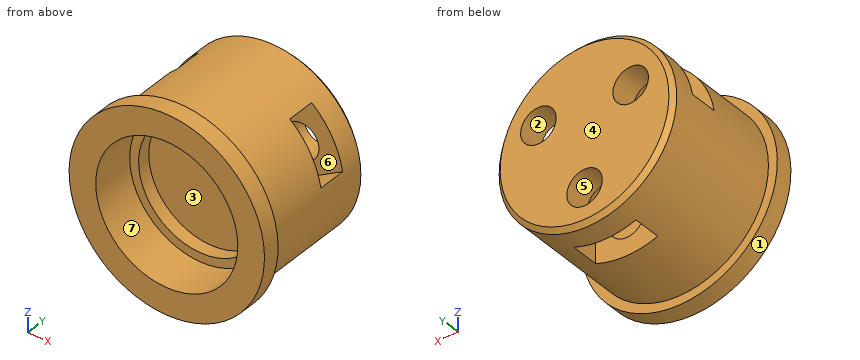
from build123d import *

# Parameters (mm, degrees)
SKETCH1_R           = 10
BOSS_EXTRUDE1_DEPTH = 16
SKETCH2_R           = 11
SKETCH2_R_2         = 10
BOSS_EXTRUDE2_DEPTH = 2
SKETCH3_R           = 8
CUT_EXTRUDE1_DEPTH  = 6.5
SKETCH4_R           = 2
CUT_EXTRUDE2_DEPTH  = 6.5
CUT_EXTRUDE3_START  = -3
SKETCH5_R           = 2
CUT_EXTRUDE3_DEPTH  = 3.2
BOSS_EXTRUDE3_START = -5
SKETCH6_R           = 8
SKETCH6_R_2         = 7
BOSS_EXTRUDE3_DEPTH = 1.5
CHAMFER1_SIZE       = 0.5


with BuildPart() as part:
    # Sketch1 → Boss-Extrude1 (new body)
    with BuildSketch(Plane(origin=(0, 0, 0), x_dir=(1, 0, 0), z_dir=(0, 1, 0))):
        with Locations(Location((0, 0, 0), (0, 0, 270))):
            Circle(SKETCH1_R)
    extrude(amount=BOSS_EXTRUDE1_DEPTH)

    # Sketch2 → Boss-Extrude2 (add)
    with BuildSketch(Plane.XZ):
        with Locations(Location((0, 0, 0), (0, 0, 270))):
            Circle(SKETCH2_R)
        with Locations(Location((0, 0, 0), (0, 0, 270))):
            Circle(SKETCH2_R_2, mode=Mode.SUBTRACT)
    extrude(amount=-BOSS_EXTRUDE2_DEPTH)

    # Sketch3 → Cut-Extrude1 (cut)
    with BuildSketch(Plane.XZ):
        with Locations(Location((0, 0, 0), (0, 0, 270))):
            Circle(SKETCH3_R)
    extrude(amount=-CUT_EXTRUDE1_DEPTH, mode=Mode.SUBTRACT)

    # Sketch4 → Cut-Extrude2 (cut)
    with BuildSketch(Plane(origin=(0, 16, 0), x_dir=(1, 0, 0), z_dir=(0, 1, 0))):
        with Locations(Location((0, 6, 0), (0, 0, 270))):
            Circle(SKETCH4_R)
        with Locations(Location((5.196152423, -3, 0), (0, 0, 270))):
            Circle(SKETCH4_R)
        with Locations(Location((-5.196152423, -3, 0), (0, 0, 270))):
            Circle(SKETCH4_R)
    extrude(amount=-CUT_EXTRUDE2_DEPTH, mode=Mode.SUBTRACT)

    # Sketch5 → Cut-Extrude3 (cut)
    # profile 1 of 3: a face of its own
    with BuildSketch(Plane(origin=(0, 16, 0), x_dir=(1, 0, 0), z_dir=(0, 1, 0)).offset(CUT_EXTRUDE3_START)):
        with BuildLine():
            Line((-3.5, 9.367496998), (-3.5, 3.979274058))
            Line((-3.5, 3.979274058), (0, 1.958548116))
            Line((0, 1.958548116), (3.5, 3.979274058))
            Line((3.5, 3.979274058), (3.5, 9.367496998))
            ThreePointArc((3.5, 9.367496998), (0, 10), (-3.5, 9.367496998))
        make_face()
        with Locations(Location((0, 6, 0), (0, 0, 270))):
            Circle(SKETCH5_R, mode=Mode.SUBTRACT)
    # profile 2 of 3: a face of its own
    with BuildSketch(Plane(origin=(0, 16, 0), x_dir=(1, 0, 0), z_dir=(0, 1, 0)).offset(CUT_EXTRUDE3_START)):
        with BuildLine():
            ThreePointArc((-9.86249037, -1.652659586), (-8.660254038, -5), (-6.36249037, -7.714837412))
            Line((-6.36249037, -7.714837412), (-1.696152423, -5.020725942))
            Line((-1.696152423, -5.020725942), (-1.696152423, -0.979274058))
            Line((-1.696152423, -0.979274058), (-5.196152423, 1.041451884))
            Line((-5.196152423, 1.041451884), (-9.86249037, -1.652659586))
        make_face()
        with Locations(Location((-5.196152423, -3, 0), (0, 0, 270))):
            Circle(SKETCH5_R, mode=Mode.SUBTRACT)
    # profile 3 of 3: a face of its own
    with BuildSketch(Plane(origin=(0, 16, 0), x_dir=(1, 0, 0), z_dir=(0, 1, 0)).offset(CUT_EXTRUDE3_START)):
        with BuildLine():
            Line((9.86249037, -1.652659586), (5.196152423, 1.041451884))
            Line((5.196152423, 1.041451884), (1.696152423, -0.979274058))
            Line((1.696152423, -0.979274058), (1.696152423, -5.020725942))
            Line((1.696152423, -5.020725942), (6.36249037, -7.714837412))
            ThreePointArc((6.36249037, -7.714837412), (8.660254038, -5), (9.86249037, -1.652659586))
        make_face()
        with Locations(Location((5.196152423, -3, 0), (0, 0, 270))):
            Circle(SKETCH5_R, mode=Mode.SUBTRACT)
    extrude(amount=-CUT_EXTRUDE3_DEPTH, mode=Mode.SUBTRACT)

    # Sketch6 → Boss-Extrude3 (add)
    with BuildSketch(Plane.XZ.offset(BOSS_EXTRUDE3_START)):
        with Locations(Location((0, 0, 0), (0, 0, 270))):
            Circle(SKETCH6_R)
        with Locations(Location((0, 0, 0), (0, 0, 270))):
            Circle(SKETCH6_R_2, mode=Mode.SUBTRACT)
    extrude(amount=-BOSS_EXTRUDE3_DEPTH)

    # Chamfer1
    chamfer1_edges = [part.edges().sort_by_distance(p)[0] for p in [
        (0, 16, -10),
    ]]
    chamfer(chamfer1_edges, length=CHAMFER1_SIZE)


solid = part.part
For this review, take the finished solid that the model builds, in its own axes (mm). Face numbers are marked on the shaded views. A direction names the side the tool comes from. Coordinates: 2 decimals unless noted, no trailing zeros. Loops run counter-clockwise (first coordinate to the right, second up) from the corner with the lowest first, then second, coordinate; pieces in that order, holes last. Notation, with made-up numbers: (76, 30.25) - (110, 30.25) arc R30 cw to (110, 64.25) - close; hole circle Ø9 at (-5, 67). An arc over 180 degrees is marked (long way). Return JSON: item names as keys, results as strings.
Item 1: Mouldability with a two-part tool opening along Z and no side actions: class the marked faces 1, 2, 3 and 4 as pulls with the +Z half, pulls with the -Z half, needs draft (parallel to the pull), parting line crosses it, or undercut.
Determined:
{"face 1": "parting line crosses it", "face 2": "undercut", "face 3": "undercut", "face 4": "needs draft"}
Item 2: For line 1 (Y direction, x = 3.75, z = 5.5); line 2 (X direction, y = 13.5, z = 3); line 3 (X direction, y = 3.7, z = 0), list the stretches that pass through material, from the lowest coordinate up.
Determined:
{"line 1": "y = 6.5 to 9.8, 13 to 16", "line 2": "x = -9.54 to -7.2, -3.2 to 3.2, 7.2 to 9.54", "line 3": "x = -10 to -8, 8 to 10"}
Item 3: For the marked faces 5, 6 and 7, list the 3-axis set-ups (+Z, -Z, +X, -X, +Y, -Y) from which the entire face can be reached by the end or side of a thin tool; tool diameter is ignored.
Determined:
{"face 5": "+Y", "face 6": "none", "face 7": "-Y"}
Item 4: Take a section at B-B (y = 12.25). Give the boundary of the cut face in (x, z), then the cut area to 3 significant figures.
Determined:
{"outline": "(-9.86, 1.65) arc R10 ccw to (-3.5, -9.37) - (-3.5, -3.98) - (0, -1.96) - (3.5, -3.98) - (3.5, -9.37) arc R10 ccw to (9.86, 1.65) - (5.2, -1.04) - (1.7, 0.98) - (1.7, 5.02) - (6.36, 7.71) arc R10 ccw to (-6.36, 7.71) - (-1.7, 5.02) - (-1.7, 0.98) - (-5.2, -1.04) - close", "area": "171 mm2"}
Item 5: Take a section at D-D (z = 4.5). State how many separate pieces and enclosed holes the cut face has, then the cut area to 3 significant figures.
Determined:
{"separate pieces": "3", "enclosed holes": "0", "area": "144 mm2"}
Item 6: Take a section at C-C (y = 3). Give the boundary of the cut face in (x, z).
Determined:
{"outline": "circle Ø20 at (0, 0); hole circle Ø16 at (0, 0)"}
Item 7: Insertion check: pin 1 (2.5 mm diameter, centred on y = 10.5, z = -6.5, fed in from +X); pin 2 (4 mm diameter, centred on y = 13.5, z = -3, fed in from +X); pin 3 (3 mm diameter, centred on x = 4, z = 2, fed in from -Y). Each pin has a flat end and moves straight along its axis. Give the tip position at first contact, or say it passes through.
Determined:
{"pin 1": "stops at x = 8.51", "pin 2": "stops at x = 9.95", "pin 3": "stops at y = 6.5"}
Item 8: Take a section at A-A (z = 0). Give the boundary of the cut face in (x, y).
Determined:
{"outline": "(-11, 0) - (-8, 0) - (-8, 5) - (-7, 5) - (-7, 6.5) - (7, 6.5) - (7, 5) - (8, 5) - (8, 0) - (11, 0) - (11, 2) - (10, 2) - (10, 15.5) - (9.5, 16) - (-9.5, 16) - (-10, 15.5) - (-10, 2) - (-11, 2) - close; hole (-7, 9.8) - (-3.39, 9.8) - (-3.39, 13) - (-7, 13) - close; hole (3.39, 9.8) - (7, 9.8) - (7, 13) - (3.39, 13) - close"}
